For this review, take the finished solid that the model builds, in its own axes (mm). Round coordinates to 2 decimals unless told otherwise and drop trailing zeros. Loops run counter-clockwise (first coordinate to the right, second up) from the corner with the lowest first, then second, coordinate; pieces in that order, holes last.
1. Clearance check with flat-ended pins moving along their axes: pin 1 Ø1.5 at (y, z) = (112, 1) entering from -X; pin 2 Ø1.5 at (x, z) = (85, 1.5) entering from -Y; pin 3 Ø1.5 at (y, z) = (-1, 1.5) entering from +X. State where each tip first meets the part, or that it passes through.
2. Consider section A-A on x = 47.5. State the section outline as (y, z) points.
3. To check wall thickness, follow line 1 along Y through (x, z) = (87, 2.75). State the ranges of the line that lie inside material, in increasing order.
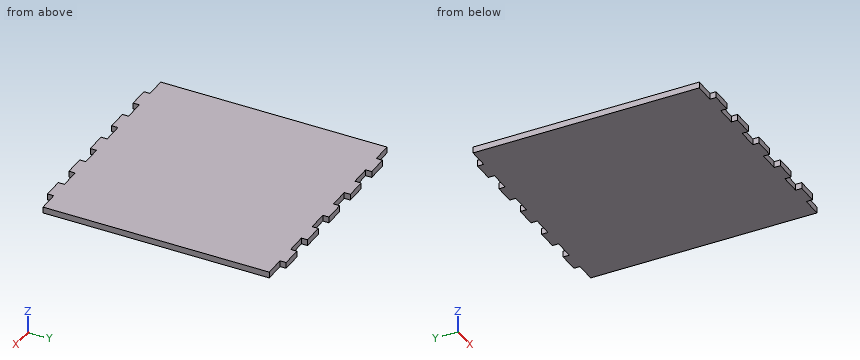
Autodesk Inventor part; units mm, degrees
ref_plane "YZ Plane" through (0, 0, 0) normal (1, 0, 0) x (0, 1, 0)
ref_plane "XZ Plane" through (0, 0, 0) normal (0, 1, 0) x (-1, 0, 0)
ref_plane "XY Plane" through (0, 0, 0) normal (0, 0, 1) x (1, 0, 0)
sketch "Sketch1" plane through (0, 0, 0) normal (0, 0, 1) x (1, 0, 0)
  line L0 (0, 0) -> (110, 0)
  line L1 (110, 0) -> (110, 110)
  line L2 (110, 110) -> (0, 110)
  line L3 (0, 110) -> (0, 0)
  dimension "d0" = 110
  dimension "d1" = 110
extrude "Extrusion1" add sketch "Sketch1" along normal blind 3
sketch "Sketch2" plane through (0, 0, 3) normal (0, 0, 1) x (1, 0, 0)
  line L0 (110, 110) -> (0, 110)
  line L1 (10, 110) -> (20, 110)
  line L2 (20, 110) -> (20, 113)
  line L3 (20, 113) -> (10, 113)
  line L4 (10, 113) -> (10, 110)
  line L5 (30, 110) -> (40, 110)
  line L6 (40, 110) -> (40, 113)
  line L7 (40, 113) -> (30, 113)
  line L8 (30, 113) -> (30, 110)
  line L9 (50, 110) -> (60, 110)
  line L10 (60, 110) -> (60, 113)
  line L11 (60, 113) -> (50, 113)
  line L12 (50, 113) -> (50, 110)
  line L13 (70, 110) -> (80, 110)
  line L14 (80, 110) -> (80, 113)
  line L15 (80, 113) -> (70, 113)
  line L16 (70, 113) -> (70, 110)
  line L17 (90, 110) -> (100, 110)
  line L18 (100, 110) -> (100, 113)
  line L19 (100, 113) -> (90, 113)
  line L20 (90, 113) -> (90, 110)
  line L21 (0, 110) -> (0, 0)
  line L22 (10, -3) -> (20, -3)
  line L23 (20, -3) -> (20, 0)
  line L24 (20, 0) -> (10, 0)
  line L25 (10, 0) -> (10, -3)
  line L26 (30, -3) -> (40, -3)
  line L27 (40, -3) -> (40, 0)
  line L28 (40, 0) -> (30, 0)
  line L29 (30, 0) -> (30, -3)
  line L30 (50, -3) -> (60, -3)
  line L31 (60, -3) -> (60, 0)
  line L32 (60, 0) -> (50, 0)
  line L33 (50, 0) -> (50, -3)
  line L34 (70, -3) -> (80, -3)
  line L35 (80, -3) -> (80, 0)
  line L36 (80, 0) -> (70, 0)
  line L37 (70, 0) -> (70, -3)
  line L38 (90, -3) -> (100, -3)
  line L39 (100, -3) -> (100, 0)
  line L40 (100, 0) -> (90, 0)
  line L41 (90, 0) -> (90, -3)
  dimension "d4" = 10
  dimension "d5" = 3
  dimension "d6" = 10
  dimension "d9" = 20
  dimension "d12" = 113
extrude "Extrusion2" add sketch "Sketch2" against normal blind 3
sketch "Sketch3" plane through (0, 0, 3) normal (0, 0, 1) x (1, 0, 0)
  point P0 (0, 0)
properties part number "Techopantalla"
Resolved:
1. pin 1: stops at x = 10
1. pin 2: stops at y = 0
1. pin 3: stops at x = 100
2. outline: (0, 0) - (110, 0) - (110, 3) - (0, 3) - close
3. line 1: y = 0 to 110
